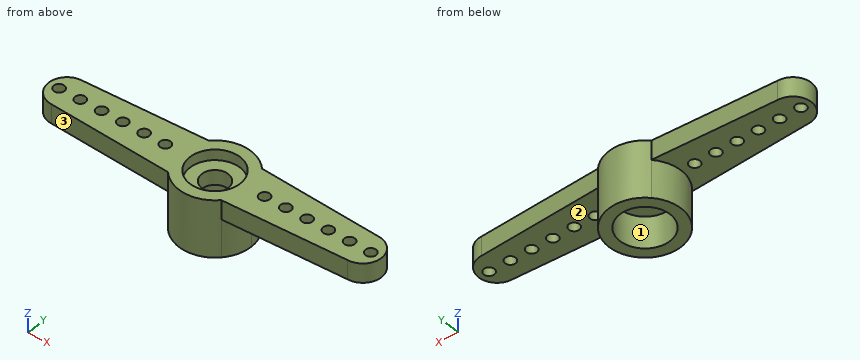
from build123d import *

# Parameters (mm, degrees)
F1_DEPTH = 0.91
F3_DEPTH = 5.4
F4_R     = 2.375
F5_DEPTH = 1
F6_R     = 2.375
F7_DEPTH = 3
F9_D     = 2.5
F11_D    = 1


with BuildPart() as f1:
    # F0 (on Top) → F1 (new body, symmetric)
    with BuildSketch(Plane.XY):
        with BuildLine():
            Line((-13.92, -1.75), (-13.92, 1.75))
            ThreePointArc((-13.92, 1.75), (-15.67, 0), (-13.92, -1.75))
        make_face()
        with BuildLine():
            ThreePointArc((-13.92, -1.75), (-12.6825631329, -1.2374368671), (-12.17, 0))
            ThreePointArc((-12.17, 0), (-12.6825631329, 1.2374368671), (-13.92, 1.75))
            Line((-13.92, 1.75), (-13.92, -1.75))
        make_face()
        with BuildLine():
            ThreePointArc((-13.92, 1.75), (-12.6825631329, 1.2374368671), (-12.17, 0))
            ThreePointArc((-12.17, 0), (-12.6825631329, -1.2374368671), (-13.92, -1.75))
            Line((-13.92, -1.75), (0, -2.45))
            Line((0, -2.45), (0, 2.45))
            Line((0, 2.45), (-13.92, 1.75))
        make_face()
        with BuildLine():
            Line((13.92, 1.75), (0, 2.45))
            Line((0, 2.45), (0, -2.45))
            Line((0, -2.45), (13.92, -1.75))
            ThreePointArc((13.92, -1.75), (12.17, 0), (13.92, 1.75))
        make_face()
        with BuildLine():
            Line((13.92, -1.75), (13.92, 1.75))
            ThreePointArc((13.92, 1.75), (12.17, 0), (13.92, -1.75))
        make_face()
        with BuildLine():
            ThreePointArc((15.67, 0), (15.1574368671, 1.2374368671), (13.92, 1.75))
            Line((13.92, 1.75), (13.92, -1.75))
            ThreePointArc((13.92, -1.75), (15.1574368671, -1.2374368671), (15.67, 0))
        make_face()
    extrude(amount=F1_DEPTH, both=True)

    # F2 (on face) → F3 (join)
    with BuildSketch(Plane.XY.offset(0.91)):
        with BuildLine():
            Line((0, 2.45), (2.5092377818, 2.3238170656))
            ThreePointArc((2.5092377818, 2.3238170656), (0, 3.42), (-2.5092377818, 2.3238170656))
            Line((-2.5092377818, 2.3238170656), (0, 2.45))
        make_face()
        with BuildLine():
            ThreePointArc((2.5092377818, -2.3238170656), (3.1841791104, -1.2479596921), (3.42, 0))
            ThreePointArc((3.42, 0), (3.1841791104, 1.2479596921), (2.5092377818, 2.3238170656))
            Line((2.5092377818, 2.3238170656), (0, 2.45))
            Line((0, 2.45), (-2.5092377818, 2.3238170656))
            ThreePointArc((-2.5092377818, 2.3238170656), (-3.42, 0), (-2.5092377818, -2.3238170656))
            Line((-2.5092377818, -2.3238170656), (0, -2.45))
            Line((0, -2.45), (2.5092377818, -2.3238170656))
        make_face()
        with BuildLine():
            ThreePointArc((-2.5092377818, -2.3238170656), (0, -3.42), (2.5092377818, -2.3238170656))
            Line((2.5092377818, -2.3238170656), (0, -2.45))
            Line((0, -2.45), (-2.5092377818, -2.3238170656))
        make_face()
    extrude(amount=-F3_DEPTH)

    # F4 (on face) → F5 (cut)
    with BuildSketch(Plane.XY.offset(0.91)):
        Circle(F4_R)
    extrude(amount=-F5_DEPTH, mode=Mode.SUBTRACT)

    # F6 (on face) → F7 (cut)
    with BuildSketch(Plane(origin=(0, 0, -4.49), x_dir=(1, 0, 0), z_dir=(0, 0, -1))):
        Circle(F6_R)
    extrude(amount=-F7_DEPTH, mode=Mode.SUBTRACT)

    # F9 (through all)
    with Locations(Plane.XY.offset(-0.09)):
        with Locations((0, 0)):
            Hole(F9_D / 2)

    # F11 (through all)
    with Locations(Plane.XY.offset(0.91)):
        with Locations((-14.67, 0), (-12.67, 0), (-10.67, 0), (-8.67, 0), (-6.67, 0), (-4.67, 0), (4.67, 0), (6.67, 0), (8.67, 0), (10.67, 0), (12.67, 0), (14.67, 0)):
            Hole(F11_D / 2)


solid = f1.part
Geometry check sheet. Reference: the model listing, model coordinates, mm. Face numbers are marked on the shaded views. Round coordinates to 2 decimals unless told otherwise and drop trailing zeros. Order: outer loops, then holes, each group sorted by start corner. A loop starts at its lowest first (then second) coordinate and runs counter-clockwise, first axis right, second up. Notation, with made-up numbers: (-8, -31) - (7, -31) arc R16 cw to (7, -3) - close; hole circle Ø10 at (-22.75, 22.25). An arc over 180 degrees is marked (long way). One line per question, with ' | ' between items. Start each with the question number.
(1) Release check for a two-part mould opening along X. For the marked faces 1, 2 and 3 record: released by +X, released by -X, zero draft, split by the parting line, or undercut.
(2) Sectioned sample at D-D on x = 0.5. Record the cut outline in (y, z), and give its area (3 significant figures).
(3) Depth check by flat-ended pin: pin 1 Ø4 at (x, y) = (-1, 1) entering from +Z; pin 2 Ø1.4 at (x, y) = (-8, 0) entering from -Z; pin 3 Ø4 at (x, y) = (0, 0) entering from -Z. Enter the tip coordinate at first touch or a pass-through.
(4) Sectioned sample at B-B on z = -3.6. Record the cut outline in (x, y) (3 decimals).
(5) Sectioned sample at C-C on x = -12.67. Record the cut outline in (y, z), and give its area (3 significant figures).
(6) Thickness scan on L1, parallel to Y at x = 0, z = -3.8 (3 decimals); L2, parallel to Z at x = -3.5, y = 2; L3, parallel to Y at x = -4.67, z = 0.2. Record the ranges inside material, lowest first. Write a range as [from, to].
(7) Sectioned sample at A-A on x = 10.67. Record the cut outline in (y, z), and give its area (3 significant figures).
Conclusion:
1) face 1: undercut | face 2: zero draft | face 3: released by -X
2) outline: (-3.38, -4.49) - (-2.32, -4.49) - (-2.32, -1.49) - (-1.15, -1.49) - (-1.15, -0.09) - (-2.32, -0.09) - (-2.32, 0.91) - (-3.38, 0.91) - close; (1.15, -1.49) - (2.32, -1.49) - (2.32, -4.49) - (3.38, -4.49) - (3.38, 0.91) - (2.32, 0.91) - (2.32, -0.09) - (1.15, -0.09) - close | area: 14.8 mm2
3) pin 1: stops at z = 0.91 | pin 2: stops at z = -0.91 | pin 3: stops at z = -1.49
4) outline: circle Ø6.84 at (0, 0); hole circle Ø4.75 at (0, 0)
5) outline: (-1.81, -0.91) - (-0.5, -0.91) - (-0.5, 0.91) - (-1.81, 0.91) - close; (0.5, -0.91) - (1.81, -0.91) - (1.81, 0.91) - (0.5, 0.91) - close | area: 4.78 mm2
6) L1: y = [-3.42, -2.375], [2.375, 3.42] | L2: z = [-0.91, 0.91] | L3: y = [-2.22, -0.5], [0.5, 2.22]
7) outline: (-1.91, -0.91) - (-0.5, -0.91) - (-0.5, 0.91) - (-1.91, 0.91) - close; (0.5, -0.91) - (1.91, -0.91) - (1.91, 0.91) - (0.5, 0.91) - close | area: 5.14 mm2
